```python
from build123d import *


with BuildPart() as part:
    # Эскиз1 → Повернуть1 (revolve)
    with BuildSketch(Plane.XY):
        with BuildLine():
            Line((0.6, 36), (12, 36))
            Line((12, 36), (12, 34.561))
            Line((12, 34.561), (15, 34.561))
            Line((15, 34.561), (15, 25.6))
            ThreePointArc((15, 25.6), (14.824264069, 25.175735931), (14.4, 25))
            Line((14.4, 25), (0.1, 25))
            Line((0.1, 25), (0.1, 31.374))
            Line((0.1, 31.374), (0, 31.374))
            Line((0, 31.374), (0, 35.4))
            ThreePointArc((0, 35.4), (0.175735931, 35.824264069), (0.6, 36))
        make_face()
    revolve(axis=Axis((-1000, 0, 0), (1, 0, 0)))


solid = part.part
```
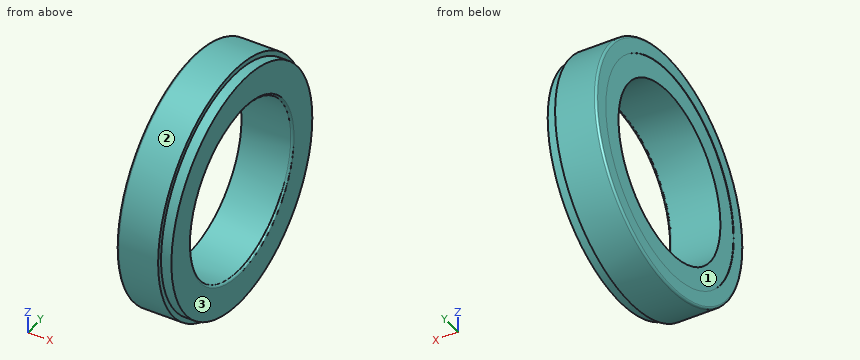
Geometry check sheet. Reference: the model listing, model coordinates, mm. Face numbers are marked on the shaded views. Give positions to 0.01 mm unless a question says otherwise; leave off trailing zeros. Loops run counter-clockwise (first coordinate to the right, second up) from the corner with the lowest first, then second, coordinate; pieces in that order, holes last. Notation, with made-up numbers: M 10.25,5 L 42.25,5 A10 ccw 42.25,20 Z; hole C 71,67.25 d5. An arc over 180 degrees is marked long. Answer as CSV lines item,"result".
Item 1: Material ranges on line 1 (Z direction, x = 9.25, y = 0); line 2 (X direction, y = 1, z = 30.5); line 3 (Z direction, x = 12.75, y = 5), recorded low to high.
Values:
line 1,"z = -36 to -25, 25 to 36"
line 2,"x = 0.1 to 15"
line 3,"z = -34.2 to -24.49, 24.49 to 34.2"
Item 2: Cross-section at D-D on x = 3.5. Record the cut outline in (y, z).
Values:
outline,"C 0,0 d72; hole C 0,0 d50"
Item 3: Cross-section at A-A on z = 0. Record the cut outline in (x, y).
Values:
outline,"M 0,-35.4 A0.6 ccw 0.6,-36 L 12,-36 L 12,-34.56 L 15,-34.56 L 15,-25.6 A0.6 ccw 14.4,-25 L 0.1,-25 L 0.1,-31.37 L 0,-31.37 Z; M 0,31.37 L 0.1,31.37 L 0.1,25 L 14.4,25 A0.6 ccw 15,25.6 L 15,34.56 L 12,34.56 L 12,36 L 0.6,36 A0.6 ccw 0,35.4 Z"
Item 4: Release check for a two-part mould opening along Y. For the marked faces 1, 2 and 3 record: pulls with the +Y half, pulls with the -Y half, needs draft (parallel to the pull), parting line crosses it, or undercut.
Values:
face 1,"undercut"
face 2,"parting line crosses it"
face 3,"needs draft"
Item 5: Depth check by flat-ended pin: P1, Ø4, axis at x = 8, y = -16.5, coming from the -Z side; P2, Ø4, axis at x = 9.5, z = -23.5, coming from the +Y side; P3, Ø8, axis at x = 10, z = 19.5, coming from the -Y side. Enter the tip coordinate at first touch or a pass-through.
Values:
P1,"stops at z = -32.95"
P2,"stops at y = 28.87"
P3,"stops at y = -32.49"
Item 6: Cross-section at C-C on x = 13.5. Record the cut outline in (y, z).
Values:
outline,"C 0,0 d69.12; hole C 0,0 d50"
